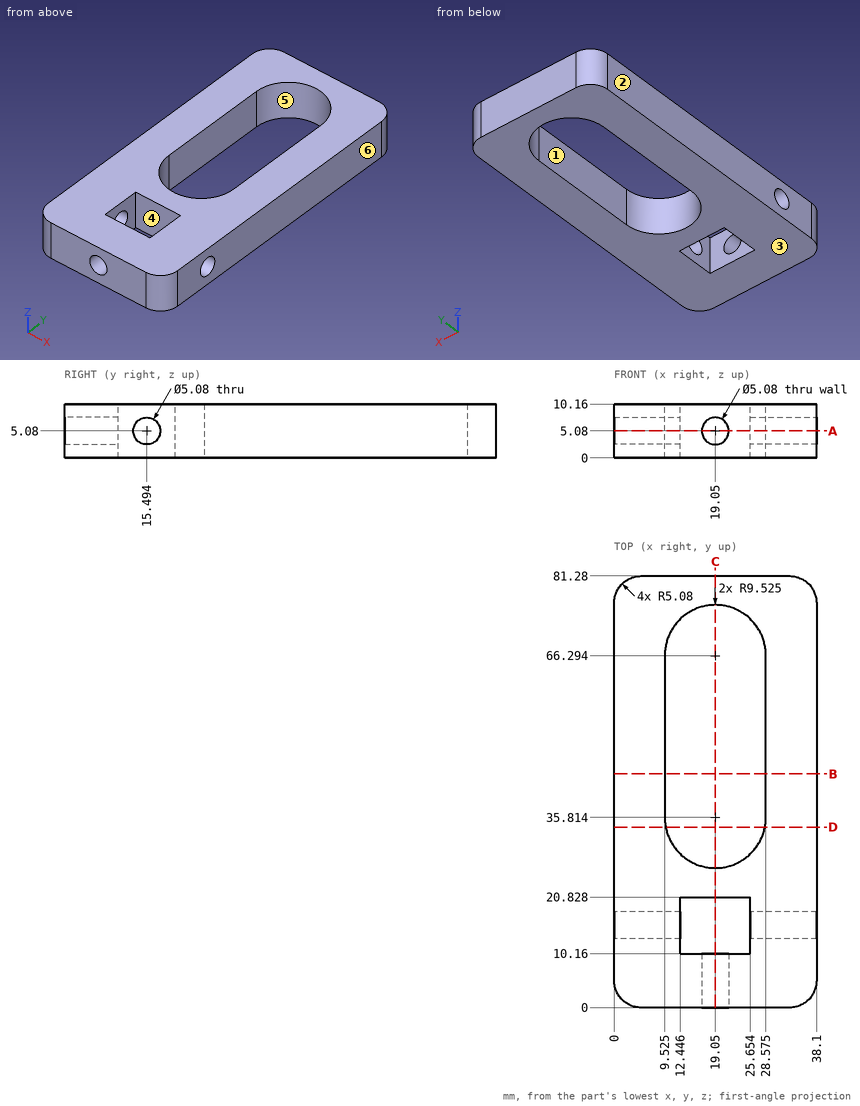
Check sheet for the drawn part. Datum: minimum x, y, z corner. Units: mm. A direction names the side the tool comes from. Coordinates: 2 decimals unless noted, no trailing zeros. Order: outer loops, then holes, each group sorted by start corner. A loop starts at its lowest first (then second) coordinate and runs counter-clockwise, first axis right, second up. Notation, with made-up numbers: (28, 63) -> (43, 63) arc R18 ccw to (43, 97) -> close; hole circle Ø5 at (71.25, 24). An arc over 180 degrees is marked (long way). Write each question's results on one line, items separated by ' | '. Start each with the question number.
1) Section check A-A (z = 5.08). Enter the section's corners in (x, y) (3 decimals), and give its area (3 significant figures).
2) Material ranges on line 1 along X through (y, z) = (7, 5.08); line 2 along Y through (x, z) = (12.5, 9.75); line 3 along Z through (x, y) = (19, 2), recorded low to high.
3) Section check B-B (y = 44). Enter the section's corners in (x, z) (3 decimals).
4) Section check D-D (y = 34). Enter the section's corners in (x, z), and give its area (3 significant figures).
5) Section check C-C (x = 19.05). Enter the section's corners in (y, z).
6) Draft check along X on the marked faces 1, 2, 3 and 4. Enter one of: pulls with the +X half, pulls with the -X half, needs draft (parallel to the pull), parting line crosses it, or undercut.
7) Set-up check for the marked faces 5 and 6: record each of +Z, -Z, +X, -X, +Y, -Y from which the full face is reachable in a straight line by a thin tool's end or side.
Checked values:
1) outline: (0, 5.08) arc R5.08 ccw to (5.08, 0) -> (16.51, 0) -> (16.51, 10.16) -> (12.446, 10.16) -> (12.446, 12.954) -> (0, 12.954) -> close; (0, 18.034) -> (12.446, 18.034) -> (12.446, 20.828) -> (25.654, 20.828) -> (25.654, 18.034) -> (38.1, 18.034) -> (38.1, 76.2) arc R5.08 ccw to (33.02, 81.28) -> (5.08, 81.28) arc R5.08 ccw to (0, 76.2) -> close; (21.59, 0) -> (33.02, 0) arc R5.08 ccw to (38.1, 5.08) -> (38.1, 12.954) -> (25.654, 12.954) -> (25.654, 10.16) -> (21.59, 10.16) -> close; hole (9.525, 35.814) arc R9.525 ccw to (28.575, 35.814) -> (28.575, 66.294) arc R9.525 ccw to (9.525, 66.294) -> close | area: 1,890 mm²
2) line 1: 0 to 16.51, 21.59 to 38.1 | line 2: 0 to 10.16, 20.83 to 28.9, 73.21 to 81.28 | line 3: 0 to 2.54, 7.62 to 10.16
3) outline: (0, 0) -> (9.525, 0) -> (9.525, 10.16) -> (0, 10.16) -> close; (28.575, 0) -> (38.1, 0) -> (38.1, 10.16) -> (28.575, 10.16) -> close
4) outline: (0, 0) -> (9.7, 0) -> (9.7, 10.16) -> (0, 10.16) -> close; (28.4, 0) -> (38.1, 0) -> (38.1, 10.16) -> (28.4, 10.16) -> close | area: 197 mm²
5) outline: (0, 0) -> (10.16, 0) -> (10.16, 2.54) -> (0, 2.54) -> close; (0, 7.62) -> (10.16, 7.62) -> (10.16, 10.16) -> (0, 10.16) -> close; (20.83, 0) -> (26.29, 0) -> (26.29, 10.16) -> (20.83, 10.16) -> close; (75.82, 0) -> (81.28, 0) -> (81.28, 10.16) -> (75.82, 10.16) -> close
6) face 1: undercut | face 2: pulls with the -X half | face 3: needs draft | face 4: undercut
7) face 5: +Z, -Z | face 6: +Z, -Z, +X, +Y, -Y
